Can you work these out from the model? Positions are in its coordinate system, mm. Face numbers are marked on the shaded views. A direction names the side the tool comes from. Round coordinates to 2 decimals unless told otherwise and drop trailing zeros. Loops run counter-clockwise (first coordinate to the right, second up) from the corner with the lowest first, then second, coordinate; pieces in that order, holes last.
(1) Which directions (+Z, -Z, +X, -X, +Y, -Y) give clear straight access to the entire face, cutting with the end or side of a thin tool? Please do the marked faces 4, 5, 6 and 7.
(2) Thinking about a two-plate mould opening in Z: for the marked faces 1, 2 and 3, which applies, released by +Z, released by -Z, zero draft, split by the parting line, or undercut?
(3) Will these pins go through, and if not, where does the flat tip stop? pin 1 Ø4 at (x, y) = (-8, 25) entering from -Z; pin 2 Ø18 at (x, y) = (-16.5, 14) entering from +Z; pin 3 Ø0.5 at (x, z) = (-35.5, -1) entering from -Y.
(4) I want a section at A-A on z = -107. Write out the boundary of the cut face in (x, y).
(5) If I drill on line 1 along X through (y, z) = (11, -84); line 2 along X through (y, z) = (22, -32) (1 decimal); line 3 along Z through (x, y) = (-19, 9) (1 decimal), over which ranges is the centre line in solid material (lowest first)?
(6) I want a section at B-B on y = 19.5. Write out the boundary of the cut face in (x, z) (1 decimal).
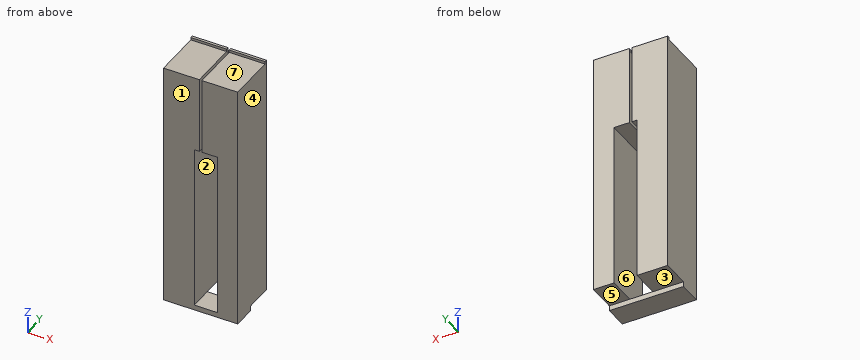
from build123d import *

# Parameters (mm, degrees)
BOSS_EXTRUDE1_DEPTH   = 31.75
BOSS_EXTRUDE1_2_DEPTH = 31.75
SKETCH2_W             = 1.5875
SKETCH2_H             = 30.1625
CUT_EXTRUDE1_DEPTH    = 47.0375
SKETCH3_W             = 3.175
SKETCH3_H             = 14.2875
BOSS_EXTRUDE2_DEPTH   = 46.0375


with BuildPart() as part:
    # Sketch1 → Boss-Extrude1 (new body)
    with BuildSketch(Plane(origin=(0, 0, 0), x_dir=(1, 0, 0), z_dir=(0, 1, 0))):
        Polygon((0, 0), (0, 152.4), (-12.7, 152.4), (-12.7, 49.2125), (-22.225, 49.2125), (-22.225, 0), align=None)
    extrude(amount=BOSS_EXTRUDE1_DEPTH)


with BuildPart() as body_2:
    # Sketch1 → Boss-Extrude1 2 (new body)
    with BuildSketch(Plane(origin=(0, 0, 0), x_dir=(1, 0, 0), z_dir=(0, 1, 0))):
        Polygon((-23.8125, 0), (-46.0375, 0), (-46.0375, 152.4), (-26.9875, 152.4), (-26.9875, 49.2125), (-23.8125, 49.2125), align=None)
    extrude(amount=BOSS_EXTRUDE1_2_DEPTH)


with BuildPart() as cut_extrude1_tool:
    # Sketch2 → Cut-Extrude1 (new body, through all)
    with BuildSketch(Plane(origin=(0, 0, 0), x_dir=(0, 0, -1), z_dir=(1, 0, 0))):
        with Locations((0.79375, 15.08125)):
            Rectangle(SKETCH2_W, SKETCH2_H)
    extrude(amount=-CUT_EXTRUDE1_DEPTH)


with BuildPart() as part_1:
    add(part.part)

    # Cut-Extrude1: cut by cut_extrude1_tool
    add(cut_extrude1_tool.part, mode=Mode.SUBTRACT)



with BuildPart() as body_2_1:
    add(body_2.part)

    # Cut-Extrude1: cut by cut_extrude1_tool
    add(cut_extrude1_tool.part, mode=Mode.SUBTRACT)


with BuildPart() as part_2:
    add(part_1.part)

    add(body_2_1.part)  # Boss-Extrude2 merges body 2
    # Sketch3 → Boss-Extrude2 (add)
    with BuildSketch(Plane(origin=(0, 0, 0), x_dir=(0, 0, -1), z_dir=(1, 0, 0))):
        with Locations((153.9875, 7.14375)):
            Rectangle(SKETCH3_W, SKETCH3_H)
    extrude(amount=-BOSS_EXTRUDE2_DEPTH)


solid = part_2.part
Filled sheet:
1. face 4: +Z, -Z, +X, +Y, -Y
1. face 5: -Z, +X, -X, +Y
1. face 6: +Y, -Y
1. face 7: +Z, +X, -X, -Y
2. face 1: zero draft
2. face 2: undercut
2. face 3: released by -Z
3. pin 1: stops at z = -152.4
3. pin 2: stops at z = -1.59
3. pin 3: stops at y = 30.16
4. outline: (-46.04, 0) - (-26.99, 0) - (-26.99, 31.75) - (-46.04, 31.75) - close; (-12.7, 0) - (0, 0) - (0, 31.75) - (-12.7, 31.75) - close
5. line 1: x = -46.04 to -26.99, -12.7 to 0
5. line 2: x = -46 to -23.8, -22.2 to 0
5. line 3: z = -155.6 to -152.4, -49.2 to -1.6
6. outline: (-46, -152.4) - (-27, -152.4) - (-27, -49.2) - (-23.8, -49.2) - (-23.8, -1.6) - (-46, -1.6) - close; (-22.2, -49.2) - (-12.7, -49.2) - (-12.7, -152.4) - (0, -152.4) - (0, -1.6) - (-22.2, -1.6) - close
